from build123d import *

# Parameters (mm, degrees)
SKETCH1_W                                         = 17.5
SKETCH1_H                                         = 10
BASE_FLANGE1_DEPTH                                = 2
EDGE_FLANGE1_DEPTH                                = 10
EDGE_FLANGE2_STRIP_W                              = 9.4732
EDGE_FLANGE2_STRIP_H                              = 2
EDGE_FLANGE2_STRIP_CUT_DEPTH                      = 10
EDGE_FLANGE2_DEPTH                                = 10
EDGE_FLANGE3_STRIP_W                              = 9.4732
EDGE_FLANGE3_STRIP_H                              = 2
EDGE_FLANGE3_STRIP_CUT_DEPTH                      = 10
EDGE_FLANGE3_DEPTH                                = 10
EDGE_FLANGE3_PROFILE_W                            = 22.5
EDGE_FLANGE3_PROFILE_H                            = 15.2634
EDGE_FLANGE3_FLAT_DEPTH                           = 2
SKETCH18_R                                        = 4
CUT_EXTRUDE2_DEPTH                                = 2
CSK_FOR_4_FLAT_HEAD_MACHINE_SCREW_100_D           = 3.2639
CSK_FOR_4_FLAT_HEAD_MACHINE_SCREW_100_DEPTH       = 2
CSK_FOR_4_FLAT_HEAD_MACHINE_SCREW_100_CSINK_D     = 5.715
CSK_FOR_4_FLAT_HEAD_MACHINE_SCREW_100_CSINK_ANGLE = 100
CSK_FOR_4_FLAT_HEAD_MACHINE_SCREW_100_TIP         = 0.980574487


# Sheet-metal steps are written as plain solids
with BuildPart() as part:
    # Sketch1 → Base-Flange1 (new body)
    with BuildSketch(Plane(origin=(0, 0, 0), x_dir=(1, 0, 0), z_dir=(0, 1, 0))):
        Rectangle(SKETCH1_W, SKETCH1_H)
    extrude(amount=BASE_FLANGE1_DEPTH)

    # Edge-Flange1 section (across the edge) → Edge-Flange1 (add)
    with BuildSketch(Plane(origin=(-5, 2, 5.7366), x_dir=(0, 0, -1), z_dir=(1, 0, 0))):
        with BuildLine():
            Line((-2, 0.7366), (-2, 62.15))
            Line((-2, 62.15), (0, 62.15))
            Line((0, 62.15), (0, 0.7366))
            ThreePointArc((0, 0.7366), (0.215745145, 0.215745145), (0.7366, 0))
            Line((0.7366, 0), (0.7366, -2))
            ThreePointArc((0.7366, -2), (-1.198468417, -1.198468417), (-2, 0.7366))
        make_face()
    extrude(amount=EDGE_FLANGE1_DEPTH)

    # Edge-Flange2 strip (across the edge) → Edge-Flange2 strip cut (cut)
    with BuildSketch(Plane(origin=(-5, 64.15, 5.7366), x_dir=(0, -1, 0), z_dir=(1, 0, 0))):
        with Locations((-2, -1)):
            Rectangle(EDGE_FLANGE2_STRIP_W, EDGE_FLANGE2_STRIP_H)
    extrude(amount=EDGE_FLANGE2_STRIP_CUT_DEPTH, mode=Mode.SUBTRACT)

    # Edge-Flange2 section (across the edge) → Edge-Flange2 (add)
    with BuildSketch(Plane(origin=(-5, 64.15, 5.7366), x_dir=(0, -1, 0), z_dir=(1, 0, 0))):
        with BuildLine():
            Line((0, 0.7366), (0, 121.685))
            Line((0, 121.685), (2, 121.685))
            Line((2, 121.685), (2, 0.7366))
            ThreePointArc((2, 0.7366), (2.215745145, 0.215745145), (2.7366, 0))
            Line((2.7366, 0), (2.7366, -2))
            ThreePointArc((2.7366, -2), (0.801531583, -1.198468417), (0, 0.7366))
        make_face()
    extrude(amount=EDGE_FLANGE2_DEPTH)

    # Edge-Flange3 strip (across the edge) → Edge-Flange3 strip cut (cut)
    with BuildSketch(Plane(origin=(-5, 62.15, -115.9484), x_dir=(0, 0, 1), z_dir=(1, 0, 0))):
        with Locations((-2, -1)):
            Rectangle(EDGE_FLANGE3_STRIP_W, EDGE_FLANGE3_STRIP_H)
    extrude(amount=EDGE_FLANGE3_STRIP_CUT_DEPTH, mode=Mode.SUBTRACT)

    # Edge-Flange3 bend section (across the edge) → Edge-Flange3 (add)
    with BuildSketch(Plane(origin=(-5, 62.15, -115.9484), x_dir=(0, 0, 1), z_dir=(1, 0, 0))):
        with BuildLine():
            Line((0, 0.7366), (2, 0.7366))
            ThreePointArc((2, 0.7366), (2.215745145, 0.215745145), (2.7366, 0))
            Line((2.7366, 0), (2.7366, -2))
            ThreePointArc((2.7366, -2), (0.801531583, -1.198468417), (0, 0.7366))
        make_face()
    extrude(amount=EDGE_FLANGE3_DEPTH)

    # Edge-Flange3 profile (on flange) → Edge-Flange3 flat (add)
    with BuildSketch(Plane(origin=(0, 62.15, -115.9484), x_dir=(1, 0, 0), z_dir=(0, 0, -1))):
        with Locations((0, 8.3683)):
            Rectangle(EDGE_FLANGE3_PROFILE_W, EDGE_FLANGE3_PROFILE_H)
    extrude(amount=-EDGE_FLANGE3_FLAT_DEPTH)

    # Sketch18 → Cut-Extrude2 (cut)
    with BuildSketch(Plane(origin=(0, 0, -115.9484), x_dir=(-1, 0, 0), z_dir=(0, 0, -1))):
        with Locations(Location((0, 53.9134, 0), (0, 0, 90))):
            Circle(SKETCH18_R)
    extrude(amount=-CUT_EXTRUDE2_DEPTH, mode=Mode.SUBTRACT)

    # CSK for #4 Flat Head Machine Screw (100)1
    with Locations(Plane.XZ):
        with Locations((4.75, 0), (-4.75, 0)):
            CounterSinkHole(CSK_FOR_4_FLAT_HEAD_MACHINE_SCREW_100_D / 2, CSK_FOR_4_FLAT_HEAD_MACHINE_SCREW_100_CSINK_D / 2, depth=CSK_FOR_4_FLAT_HEAD_MACHINE_SCREW_100_DEPTH, counter_sink_angle=CSK_FOR_4_FLAT_HEAD_MACHINE_SCREW_100_CSINK_ANGLE)
            with Locations((0, 0, -(CSK_FOR_4_FLAT_HEAD_MACHINE_SCREW_100_DEPTH + CSK_FOR_4_FLAT_HEAD_MACHINE_SCREW_100_TIP / 2))):  # 118° drill point
                Cone(0, CSK_FOR_4_FLAT_HEAD_MACHINE_SCREW_100_D / 2, CSK_FOR_4_FLAT_HEAD_MACHINE_SCREW_100_TIP, mode=Mode.SUBTRACT)


solid = part.part
Read the model definition and answer for the solid it produces. Units are mm, in the model's axes. A direction names the side the tool comes from. Round coordinates to 2 decimals unless told otherwise and drop trailing zeros. Write each loop counter-clockwise with the first axis right and the second up, starting at its lowest first coordinate (ties: lowest second). Pieces come first, ordered by that corner, then holes. Notation, with made-up numbers: (19, 60.25) - (60, 60.25) arc R24 ccw to (60, 77.25) - close; hole circle Ø9 at (32.25, 82). An arc over 180 degrees is marked (long way). One line per question, with ' | ' between items. Start each with the question number.
1. Each of these flat-tipped pins is pushed along its axis until it touches: pin 1 (4 mm diameter, centred on x = 4.75, z = 0, fed in from -Y); pin 2 (2 mm diameter, centred on x = -6.5, y = 1, fed in from +Z); pin 3 (3 mm diameter, centred on x = -6, z = -43.5, fed in from -Y). Where does it stop, or does it pass through?
2. Find the intervals of material crossed by probe 1 along X at (y, z) = (1.6, 0); probe 2 along Z at (x, y) = (2, 58); probe 3 along Z at (x, y) = (-2.25, 29.5), in increasing order. Write a range as [from, to].
3. For faces 1 (the face through (0.176, 49.917, -114.962)), 2 (the face through (-3, 50, -113.948)), 3 (the face through (-4.396, 1.521, -1.593)), 4 (the face through (0, 32, 5.737)), determine the directions among +Z, -Z, +X, -X, +Y, -Y from which every point of the face is accessible in a straight line to the end or side of a thin tool.
4. Section C-C (z = -39) is taken. Determine the outline of the cut face in (x, y).
5. Section B-B (y = 21.5) is taken. Determine the outline of the cut face in (x, z).
6. Section A-A (x = 0) is taken. Determine the outline of the cut face in (y, z), and give its area (3 significant figures).
7. For a pull along X with two mould halves and no side action, classify faces 5 (the face through (0, 64.15, -53)), 6 (the face through (3.242, 1.521, -0.625)), 7 (the face through (5, 63, -54)) as +X half, -X half, draft (parallel to the pull), parting line (faces both ways), or undercut.
Filled in:
1) pin 1: y = 0.72 | pin 2: z = 5 | pin 3: y = 62.15
2) probe 1: [-8.75, -6.38], [-3.12, 3.12], [6.38, 8.75] | probe 2: [-115.95, -113.95], [5.74, 7.74] | probe 3: [5.74, 7.74]
3) face 1: -Z | face 2: +X, -X, -Y | face 3: -Y | face 4: +X, -X
4) outline: (-5, 62.15) - (5, 62.15) - (5, 64.15) - (-5, 64.15) - close
5) outline: (-5, 5.74) - (5, 5.74) - (5, 7.74) - (-5, 7.74) - close
6) outline: (0, -5) - (2, -5) - (2, 5) arc R0.74 cw to (2.74, 5.74) - (61.41, 5.74) arc R0.74 cw to (62.15, 5) - (62.15, -113.21) arc R0.74 cw to (61.41, -113.95) - (57.91, -113.95) - (57.91, -115.95) - (61.41, -115.95) arc R2.74 ccw to (64.15, -113.21) - (64.15, 5) arc R2.74 ccw to (61.41, 7.74) - (2.74, 7.74) arc R2.74 ccw to (0, 5) - close; (46.15, -115.95) - (49.91, -115.95) - (49.91, -113.95) - (46.15, -113.95) - close | area: 405 mm²
7) face 5: draft | face 6: undercut | face 7: +X half
